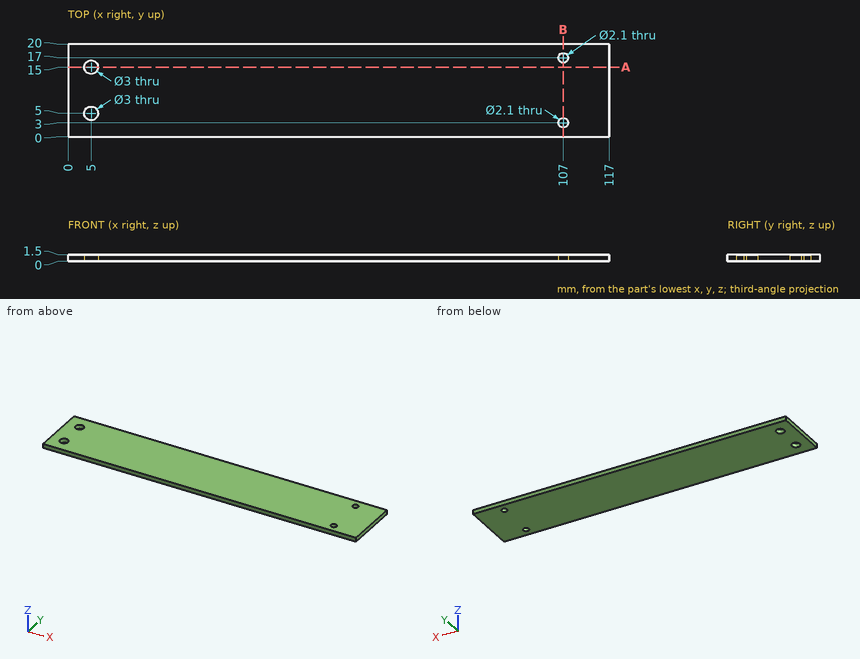
The figure shows three views and two pictorial views of one solid part (mm, origin at its lowest corner). Answer the questions. Give positions to 0.01 mm unless a question says otherwise; leave off trailing zeros. Write each loop counter-clockwise with the first axis right and the second up, starting at its lowest first coordinate (ties: lowest second). Pieces come first, ordered by that corner, then holes. Notation, with made-up numbers: (2.25, 53) - (38.25, 53) arc R11 cw to (38.25, 60) - close; hole circle Ø10 at (57.5, 18). An arc over 180 degrees is marked (long way). Return JSON: item names as keys, results as strings.
Q1. Consider line 1 along Y through (x, z) = (5, 0.95); line 2 along X through (y, z) = (5.25, 1.2); line 3 along Y through (x, z) = (107, 0.95). Determine where each line is inside the solid, lowest interval first. Write a range as [from, to].
Reply:
{"line 1": "[0, 3.5], [6.5, 13.5], [16.5, 20]", "line 2": "[0, 3.52], [6.48, 117]", "line 3": "[0, 1.95], [4.05, 15.95], [18.05, 20]"}
Q2. A cutting plane is placed at B-B, the plane x = 107. Determine the outline of the cut face in (y, z).
Reply:
{"outline": "(0, 0) - (1.95, 0) - (1.95, 1.5) - (0, 1.5) - close; (4.05, 0) - (15.95, 0) - (15.95, 1.5) - (4.05, 1.5) - close; (18.05, 0) - (20, 0) - (20, 1.5) - (18.05, 1.5) - close"}
Q3. A cutting plane is placed at A-A, the plane y = 15. Determine the outline of the cut face in (x, z).
Reply:
{"outline": "(0, 0) - (3.5, 0) - (3.5, 1.5) - (0, 1.5) - close; (6.5, 0) - (117, 0) - (117, 1.5) - (6.5, 1.5) - close"}
Q4. Given P1, Ø2.5, axis at x = 107, y = 3, coming from the -Z side, flat-ended and moving along its own axis, determine where the tip first touches the part or whether it passes through.
Reply:
{"P1": "z = 0"}
